Answer from the drawing. Dimensions are ordinates in mm from the lowest x, y and z of the part. Give positions to 0.01 mm unless a question says otherwise; leave off trailing zeros. Write each loop counter-clockwise with the first axis right and the second up, starting at its lowest first coordinate (ties: lowest second). Pieces come first, ordered by that corner, then holes.
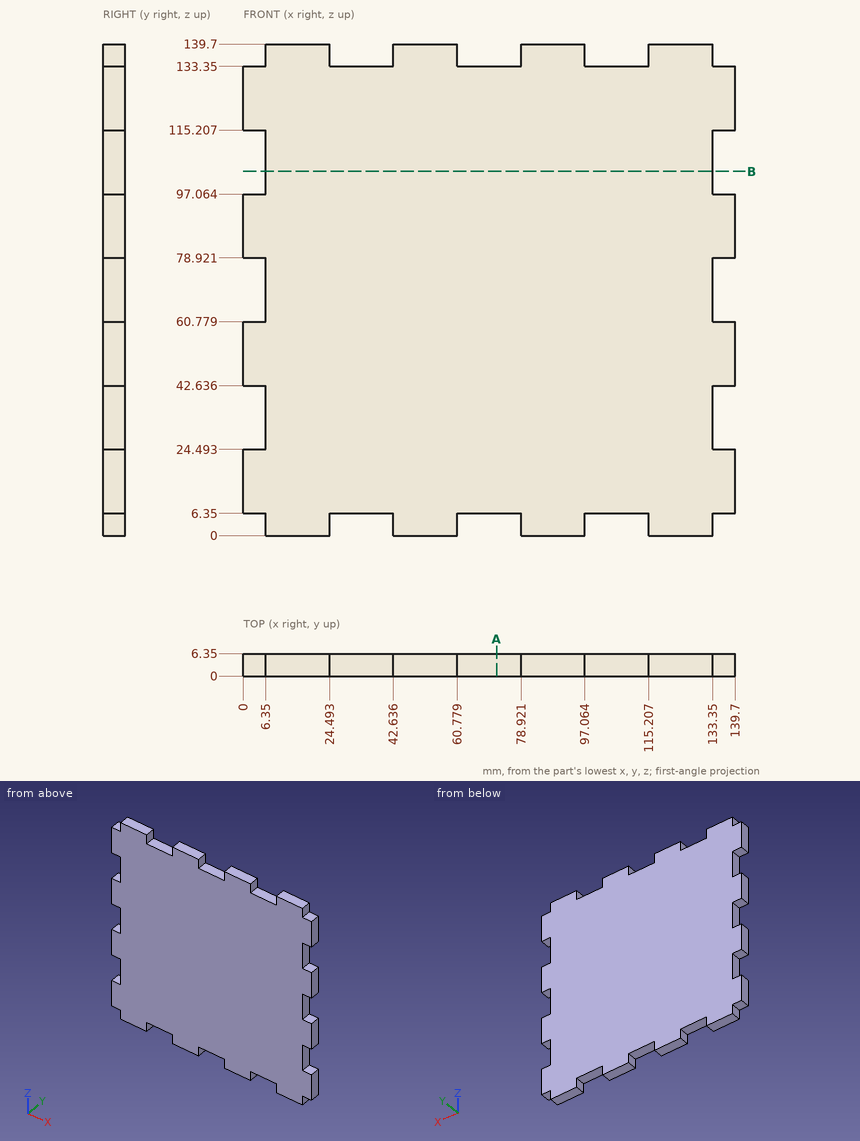
Item 1: Each of these flat-tipped pins is pushed along its axis until it touches: pin 1 Ø1.5 at (y, z) = (2, 77.5) entering from +X; pin 2 Ø3 at (x, y) = (136, 4) entering from -Z; pin 3 Ø3 at (y, z) = (3.5, 3.5) entering from -X. Where does it stop, or does it pass through?
Result set:
pin 1: stops at x = 133.35
pin 2: stops at z = 6.35
pin 3: stops at x = 6.35
Item 2: Section B-B (z = 103.5) is taken. Write down the section's boundary in (x, y).
Result set:
outline: (6.35, 0) - (133.35, 0) - (133.35, 6.35) - (6.35, 6.35) - close
Item 3: Section A-A (x = 72) is taken. Write down the section's boundary in (y, z).
Result set:
outline: (0, 6.35) - (6.35, 6.35) - (6.35, 133.35) - (0, 133.35) - close
Item 4: Find the intervals of material crossed by line 1 along Z through (x, y) = (41.5, 1.5), in increasing order.
Result set:
line 1: z = 6.35 to 133.35
